from build123d import *

# Parameters (mm, degrees)
BOSS_EXTRU_1_DEPTH = 8


with BuildPart() as part:
    # Esquisse1 → Boss.-Extru.1 (new body)
    with BuildSketch(Plane.XY):
        with BuildLine():
            Line((-48.206262386, 70.57122428), (-48.206262386, 52.692544623))
            ThreePointArc((-48.206262386, 52.692544623), (-48.206262386, 50.57122428), (-50.327582729, 50.57122428))
            Line((-50.327582729, 50.57122428), (-56.206262386, 50.57122428))
            Line((-56.206262386, 50.57122428), (-56.206262386, 10.57122428))
            Line((-56.206262386, 10.57122428), (-50.327582729, 10.57122428))
            ThreePointArc((-50.327582729, 10.57122428), (-48.206262386, 10.57122428), (-48.206262386, 8.449903936))
            Line((-48.206262386, 8.449903936), (-48.206262386, -9.42877572))
            Line((-48.206262386, -9.42877572), (37.793737614, -9.42877572))
            Line((37.793737614, -9.42877572), (37.793737614, 70.57122428))
            Line((37.793737614, 70.57122428), (29.793737614, 70.57122428))
            Line((29.793737614, 70.57122428), (29.793737614, 50.57122428))
            Line((29.793737614, 50.57122428), (21.293737614, 50.57122428))
            Line((21.293737614, 50.57122428), (21.293737614, 70.57122428))
            Line((21.293737614, 70.57122428), (-48.206262386, 70.57122428))
        make_face()
        with BuildLine():
            Line((-15.511163156, 25.07122428), (14.488836844, 25.07122428))
            ThreePointArc((14.488836844, 25.07122428), (26.988836844, 12.57122428), (14.488836844, 0.07122428))
            Line((14.488836844, 0.07122428), (-15.511163156, 0.07122428))
            ThreePointArc((-15.511163156, 0.07122428), (-28.011163156, 12.57122428), (-15.511163156, 25.07122428))
        make_face(mode=Mode.SUBTRACT)
    extrude(amount=BOSS_EXTRU_1_DEPTH)


solid = part.part
Source: CAD feature listing. Evaluate the final solid. Frame: model axes, mm. A direction names the side the tool comes from. Coordinates: 2 decimals unless noted, no trailing zeros. Loops run counter-clockwise (first coordinate to the right, second up) from the corner with the lowest first, then second, coordinate; pieces in that order, holes last. Notation, with made-up numbers: (-6, 66.25) - (40, 66.25) arc R26 cw to (40, 87.25) - close; hole circle Ø7 at (52, -29.5). An arc over 180 degrees is marked (long way). Return JSON: item names as keys, results as strings.
Q1. Section B-B, the plane x = 4. Return loops of the section in (y, z), plus the area to 3 significant figures.
Results:
{"outline": "(-9.43, 0) - (0.07, 0) - (0.07, 8) - (-9.43, 8) - close; (25.07, 0) - (70.57, 0) - (70.57, 8) - (25.07, 8) - close", "area": "440 mm2"}
Q2. Section A-A, the plane z = 5.5. Return loops of the section in (x, y), plus the area to 3 significant figures.
Results:
{"outline": "(-56.21, 10.57) - (-50.33, 10.57) arc R1.5 cw to (-48.21, 8.45) - (-48.21, -9.43) - (37.79, -9.43) - (37.79, 70.57) - (29.79, 70.57) - (29.79, 50.57) - (21.29, 50.57) - (21.29, 70.57) - (-48.21, 70.57) - (-48.21, 52.69) arc R1.5 cw to (-50.33, 50.57) - (-56.21, 50.57) - close; hole (-15.51, 0.07) - (14.49, 0.07) arc R12.5 ccw to (14.49, 25.07) - (-15.51, 25.07) arc R12.5 ccw to start", "area": "5,790 mm2"}
Q3. Material intervals for line 1 along X through (y, z) = (60, 5.5); line 2 along Y through (x, z) = (-14, 1.5); line 3 along X through (y, z) = (-0.5, 6.5), sorted ascending.
Results:
{"line 1": "-48.21 to 21.29, 29.79 to 37.79", "line 2": "-9.43 to 0.07, 25.07 to 70.57", "line 3": "-48.21 to 37.79"}
Q4. Access query for faces 5 (the flat face through (-53, 10.571, 4)), 6 (the flat face through (-48.206, 62, 4)), 7 (the cylindrical face through (26.986, 12.846, 3.944)). Directions: +Z, -Z, +X, -X, +Y, -Y. A direction counts if a zero-diameter tool reaches every point of the face in a straight line with its end or side. Return the directions, or none.
Results:
{"face 5": "+Z, -Z, -X, -Y", "face 6": "+Z, -Z, -X, +Y", "face 7": "+Z, -Z"}
Q5. Mould query, pull axis Y, two halves, no side actions, for faces 1 (the flat face through (0, 0.071, 4)), 2 (the cylindrical face through (-48.183, 50.595, 3.944)), 3 (the flat face through (37.794, 30, 4)), 4 (the flat face through (-6, -9.429, 4)). Classes: released by +Y, released by -Y, zero draft, split by the parting line, or undercut.
Results:
{"face 1": "undercut", "face 2": "undercut", "face 3": "zero draft", "face 4": "released by -Y"}
Q6. Section C-C, the plane y = 17. Return loops of the section in (x, z), plus the area to 3 significant figures.
Results:
{"outline": "(-56.21, 0) - (-27.2, 0) - (-27.2, 8) - (-56.21, 8) - close; (26.18, 0) - (37.79, 0) - (37.79, 8) - (26.18, 8) - close", "area": "325 mm2"}
Q7. Contact query for flat-ended pins moving along their axis: P1, Ø1, axis at x = 22.5, y = 57, coming from the -Z side; P2, Ø2.5, axis at x = 26, z = 5.5, coming from the +Y side. Output: stop coordinate, or through.
Results:
{"P1": "through", "P2": "y = 50.57"}
